Study the drawing (mm; zero at the part's minimum x, y, z) and answer. Give positions to 0.01 mm unless a question says otherwise; leave off trailing zeros. Loops run counter-clockwise (first coordinate to the right, second up) from the corner with the lowest first, then second, coordinate; pieces in that order, holes last. Notation, with made-up numbers: M 87.5,68.5 L 105.5,68.5 A10 ccw 105.5,79.5 Z; hole C 57.5,-35.75 d9. An arc over 180 degrees is marked long. Use one line per item in the form item = value. Start each with the question number.
1. The part is cut by section D-D (z = 11.5). Write down the section's boundary in (x, y).
2. Each of these flat-tipped pins is pushed along its axis until it touches: pin 1 Ø10 at (x, z) = (8.5, 28.5) entering from -Y (1 decimal); pin 2 Ø1.5 at (y, z) = (15, 41) entering from +X (1 decimal); pin 3 Ø3 at (y, z) = (15.5, 50.5) entering from +X (1 decimal). Where does it stop, or does it pass through?
3. Straight lines are drawn through the part: line 1 (Y direction, x = 30, z = 61); line 2 (Y direction, x = 30, z = 22); line 3 (X direction, y = 39.5, z = 42.5) (1 decimal). For each, find the intervals that lie inside material, in ascending order. Write a range as from..to.
4. The mould has two halves that part along Y. Classify the marked faces 1, 2, 3 and 4: released by +Y, released by -Y, zero draft, split by the parting line, or undercut.
5. The part is cut by section C-C (z = 61.5). Write down the section's boundary in (x, y) (1 decimal).
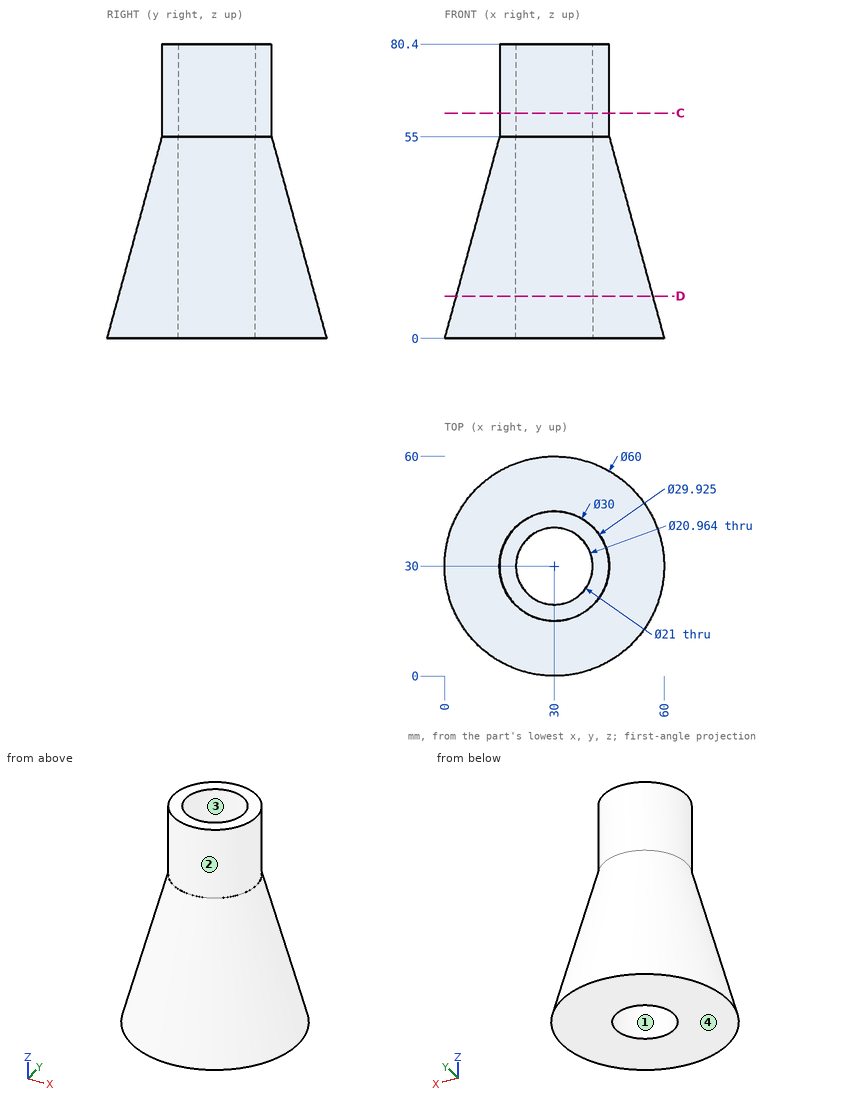
Derived:
q1.outline = C 30,30 d53.73; hole C 30,30 d21
q2.pin_1 = 14.7
q2.pin_2 = 42.3
q2.pin_3 = 39.8
q3.line_1 = 15.04..19.52, 40.48..44.96
q3.line_2 = 6..19.5, 40.5..54
q3.line_3 = 14.2..25.5, 34.5..45.8
q4.face_1 = undercut
q4.face_2 = split by the parting line
q4.face_3 = undercut
q4.face_4 = zero draft
q5.outline = C 30,30 d29.9; hole C 30,30 d21
